from build123d import *

# Parameters (mm, degrees)
BOSS_EXTRUDE1_DEPTH = 5
SKETCH2_R           = 1.6
CUT_EXTRUDE1_DEPTH  = 5
BOSS_EXTRUDE2_DEPTH = 12.5
CUT_EXTRUDE2_START  = -12.5
SKETCH4_R           = 1.6
CUT_EXTRUDE2_DEPTH  = 12.5


with BuildPart() as part:
    # Sketch1 → Boss-Extrude1 (new body)
    with BuildSketch(Plane.XY):
        Polygon((-2.374519268, 1.641642951), (-2.608964134, -1.235572533), (-0.234444865, -2.877215483), (2.374519268, -1.641642951), (2.608964134, 1.235572533), (0.234444865, 2.877215483), align=None)
    extrude(amount=BOSS_EXTRUDE1_DEPTH)

    # Sketch2 → Cut-Extrude1 (cut)
    with BuildSketch(Plane.XY.offset(5)):
        Circle(SKETCH2_R)
    extrude(amount=-CUT_EXTRUDE1_DEPTH, mode=Mode.SUBTRACT)

    # Sketch3 → Boss-Extrude2 (add)
    with BuildSketch(Plane.XY.offset(5)):
        Polygon((-0.234444865, -2.877215483), (2.374519268, -1.641642951), (2.608964134, 1.235572533), (0.234444865, 2.877215483), (-2.374519268, 1.641642951), (-2.608964134, -1.235572533), align=None)
    extrude(amount=BOSS_EXTRUDE2_DEPTH)

    # Sketch4 → Cut-Extrude2 (cut)
    with BuildSketch(Plane(origin=(0, 0, 5), x_dir=(-1, 0, 0), z_dir=(0, 0, -1)).offset(CUT_EXTRUDE2_START)):
        with Locations(Location((0, 0, 0), (0, 0, 180))):
            Circle(SKETCH4_R)
    extrude(amount=CUT_EXTRUDE2_DEPTH, mode=Mode.SUBTRACT)


solid = part.part
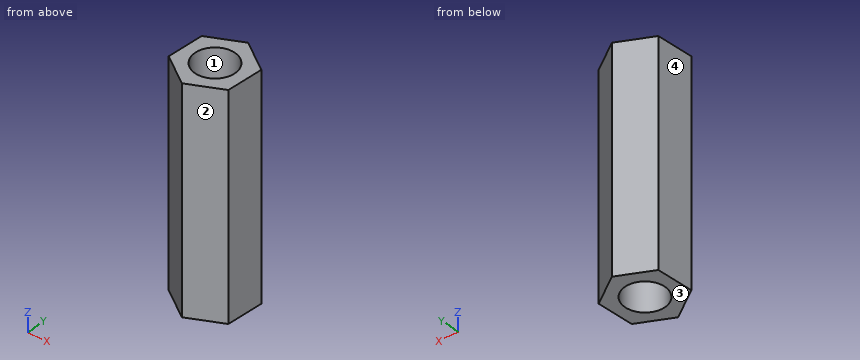
Read the model definition and answer for the solid it produces. Units are mm, in the model's axes. Face numbers are marked on the shaded views. Give positions to 0.01 mm unless a question says otherwise; leave off trailing zeros. Loops run counter-clockwise (first coordinate to the right, second up) from the corner with the lowest first, then second, coordinate; pieces in that order, holes last. Notation, with made-up numbers: (59, -10) - (64, -10) arc R19 cw to (64, -6) - close; hole circle Ø3 at (-30.75, 38.25). An arc over 180 degrees is marked (long way). Answer as CSV lines item,"result". Start each with the question number.
1) Find section C-C (x = 0.9). Write down the section's boundary in (y, z).
2) Find section A-A (z = 7.5). Write down the section's boundary in (x, y).
3) Straight lines are drawn through the part: L1, parallel to X at y = -0.95, z = 11.5; L2, parallel to Y at x = 0, z = 8; L3, parallel to X at y = 1.15, z = 12.75. For each, find the intervals that lie inside material, in ascending order. Write a range as from..to.
4) Each of these flat-tipped pins is pushed along its axis until it touches: pin 1 Ø3 at (x, y) = (0.5, -1) entering from -Z; pin 2 Ø1 at (y, z) = (-0.5, 10) entering from -X. Where does it stop, or does it pass through?
5) Find section B-B (y = 0). Write down the section's boundary in (x, z).
6) Determine the mould class of the marked faces 1, 2, 3 and 4 for opening direction X: released by +X, released by -X, zero draft, split by the parting line, or undercut.
Findings below:
1,outline,"(-2.34, 0) - (-1.32, 0) - (-1.32, 17.5) - (-2.34, 17.5) - close; (1.32, 0) - (2.42, 0) - (2.42, 17.5) - (1.32, 17.5) - close"
2,outline,"(-2.61, -1.24) - (-0.23, -2.88) - (2.37, -1.64) - (2.61, 1.24) - (0.23, 2.88) - (-2.37, 1.64) - close; hole circle Ø3.2 at (0, 0)"
3,L1,"-2.59..-1.29, 1.29..2.43"
3,L2,"-2.77..-1.6, 1.6..2.77"
3,L3,"-2.41..-1.11, 1.11..2.6"
4,pin 1,"z = 0"
4,pin 2,"x = -2.59"
5,outline,"(-2.51, 0) - (-1.6, 0) - (-1.6, 17.5) - (-2.51, 17.5) - close; (1.6, 0) - (2.51, 0) - (2.51, 17.5) - (1.6, 17.5) - close"
6,face 1,"undercut"
6,face 2,"released by +X"
6,face 3,"zero draft"
6,face 4,"released by -X"
